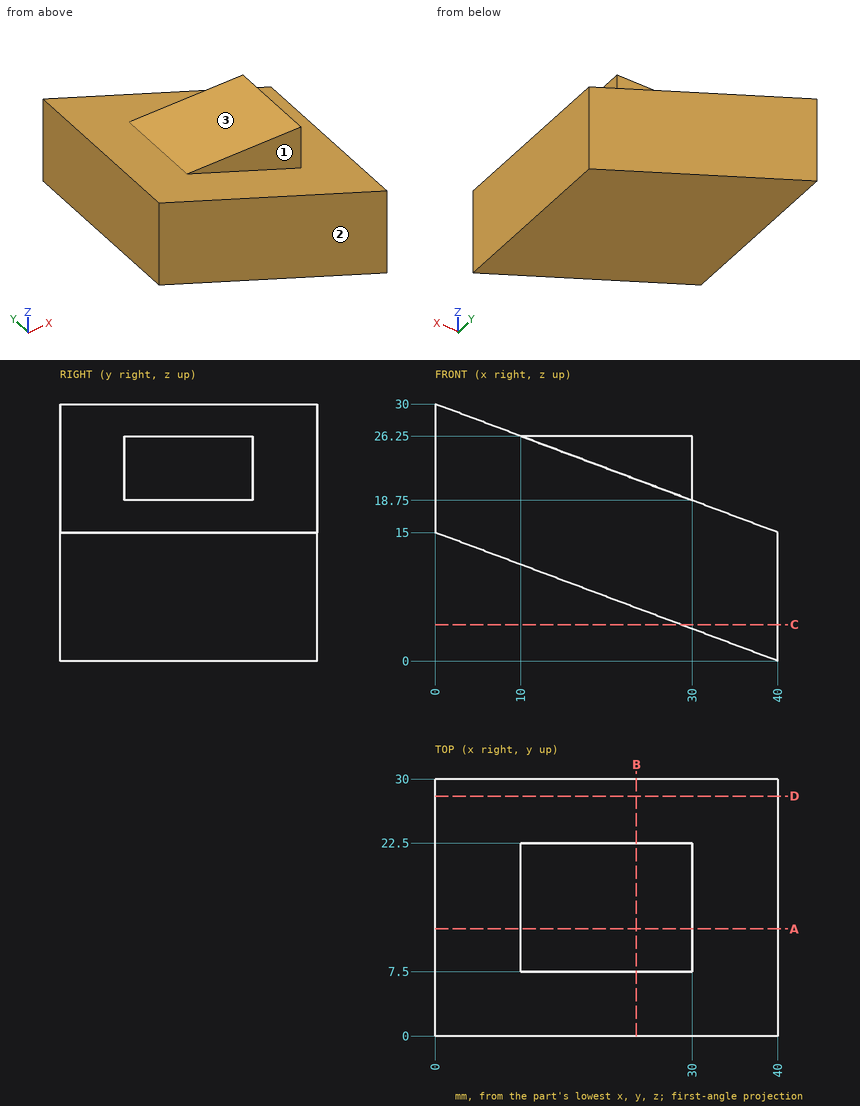
Answer from the drawing. Dimensions are ordinates in mm from the lowest x, y and z of the part. A direction names the side the tool comes from. Coordinates: 2 decimals unless noted, no trailing zeros. Write each loop counter-clockwise with the first axis right and the second up, starting at its lowest first coordinate (ties: lowest second). Pieces come first, ordered by that corner, then holes. Notation, with made-up numbers: (-25.5, 43) - (-13.5, 43) arc R16 ccw to (-13.5, 65) - close; hole circle Ø4 at (-20, 62). An arc over 180 degrees is marked (long way). Return JSON: item names as keys, results as strings. Group by question number.
Q1. Which of the six approach directions +Z, -Z, +X, -X, +Y, -Y give full straight-line access (tool end or side, diameter ignored) to the marked faces 1, 2 and 3?
Q2. The part is cut by section A-A on y = 12.5. Write down the section's boundary in (x, z).
Q3. The part is cut by section C-C on z = 4.25. Write down the section's boundary in (x, y).
Q4. The part is cut by section B-B on x = 23.5. Write down the section's boundary in (y, z), and give its area (3 significant figures).
Q5. Find the intervals of material crossed by line 1 along Y through (x, z) = (25.5, 23.5); line 2 along X through (y, z) = (20.5, 22); line 3 along Z through (x, y) = (38.5, 18.5), in increasing order. Write a range as [from, to].
Q6. Flat-ended cylindrical pins translate along their axes: pin 1 Ø8 at (y, z) = (15, 24) entering from +X; pin 2 Ø4.5 at (x, y) = (23, 13) entering from +Z; pin 3 Ø6 at (x, y) = (18.5, 3) entering from +Z. Find the tip coordinate at first contact, or state that the pin passes through.
Q7. The part is cut by section D-D on y = 28. Write down the section's boundary in (x, z), and give its area (3 significant figures).
Evaluation:
{
 "1": {"face 1": "+Z, +X, -Y", "face 2": "+Z, -Z, +X, -X, -Y", "face 3": "+Z, +X, +Y, -Y"},
 "2": {"outline": "(0, 15) - (40, 0) - (40, 15) - (30, 18.75) - (30, 26.25) - (10, 26.25) - (0, 30) - close"},
 "3": {"outline": "(28.67, 0) - (40, 0) - (40, 30) - (28.67, 30) - close"},
 "4": {"outline": "(0, 6.19) - (30, 6.19) - (30, 21.19) - (22.5, 21.19) - (22.5, 26.25) - (7.5, 26.25) - (7.5, 21.19) - (0, 21.19) - close", "area": "526 mm2"},
 "5": {"line 1": "y = [7.5, 22.5]", "line 2": "x = [0, 30]", "line 3": "z = [0.56, 15.56]"},
 "6": {"pin 1": "stops at x = 30", "pin 2": "stops at z = 26.25", "pin 3": "stops at z = 24.19"},
 "7": {"outline": "(0, 15) - (40, 0) - (40, 15) - (0, 30) - close", "area": "600 mm2"}
}
